Geometry check sheet. Reference: the model listing, model coordinates, mm. Round coordinates to 2 decimals unless told otherwise and drop trailing zeros. Write each loop counter-clockwise with the first axis right and the second up, starting at its lowest first coordinate (ties: lowest second). Pieces come first, ordered by that corner, then holes.
Item 1: Cross-section at B-B (z = 5). Enter the section's corners in (x, y), then the cut area to 3 significant figures.
Item 2: Cross-section at A-A (x = 55). Enter the section's corners in (y, z), then the cut area to 3 significant figures.
Item 3: Scan line: probe 1 along Z at (x, y) = (5, 0.3). Record every from-to range of solid material in increasing order.
Item 4: Draft check along X on faces 1 (the face through (60, 1, 30)), 2 (the face through (5, 1, 57)), 3 (the face through (53, 1, 5)), 4 (the face through (30, 1, 0)). Enter one of: pulls with the +X half, pulls with the -X half, needs draft (parallel to the pull), parting line crosses it, or undercut.
Autodesk Inventor part; units mm, degrees
ref_plane "YZ Plane" through (0, 0, 0) normal (1, 0, 0) x (0, 1, 0)
ref_plane "XZ Plane" through (0, 0, 0) normal (0, 1, 0) x (-1, 0, 0)
ref_plane "XY Plane" through (0, 0, 0) normal (0, 0, 1) x (1, 0, 0)
sketch "Sketch1" plane through (0, 0, 0) normal (0, 1, 0) x (-1, 0, 0)
  line L0 (0, 0) -> (-60, 0)
  line L1 (-60, 0) -> (-60, 60)
  line L2 (-60, 60) -> (0, 60)
  line L3 (0, 60) -> (0, 0)
  dimension "d0" = 60
  dimension "d1" = 60
extrude "Extrusion1" add sketch "Sketch1" along normal blind 1.5
sketch "Sketch2" plane through (0, 0, 0) normal (0, -1, 0) x (1, 0, 0)
  circle A0 centre (5, 5) radius 2
  circle A1 centre (5, 55) radius 2
  circle A2 centre (55, 55) radius 2
  circle A3 centre (55, 5) radius 2
  line L0 (60, 60) -> (0, 60)
  line L1 (60, 0) -> (60, 60)
  line L2 (0, 60) -> (0, 0)
  line L3 (0, 0) -> (60, 0)
  dimension "d4" = 4
  dimension "d5" = 4
  dimension "d6" = 4
  dimension "d7" = 4
  dimension "d8" = 5
  dimension "d9" = 5
  dimension "d10" = 5
  dimension "d11" = 5
  dimension "d12" = 5
  dimension "d13" = 5
  dimension "d14" = 5
  dimension "d15" = 5
extrude "Extrusion2" cut sketch "Sketch2" against normal blind 1.5 keep common part
properties part number "Deksel"
Resolved:
1. outline: (0, 0) - (3, 0) - (3, 1.5) - (0, 1.5) - close; (7, 0) - (53, 0) - (53, 1.5) - (7, 1.5) - close; (57, 0) - (60, 0) - (60, 1.5) - (57, 1.5) - close
1. area: 78.0 mm2
2. outline: (0, 0) - (1.5, 0) - (1.5, 3) - (0, 3) - close; (0, 7) - (1.5, 7) - (1.5, 53) - (0, 53) - close; (0, 57) - (1.5, 57) - (1.5, 60) - (0, 60) - close
2. area: 78.0 mm2
3. probe 1: z = 0 to 3, 7 to 53, 57 to 60
4. face 1: pulls with the +X half
4. face 2: undercut
4. face 3: undercut
4. face 4: needs draft
